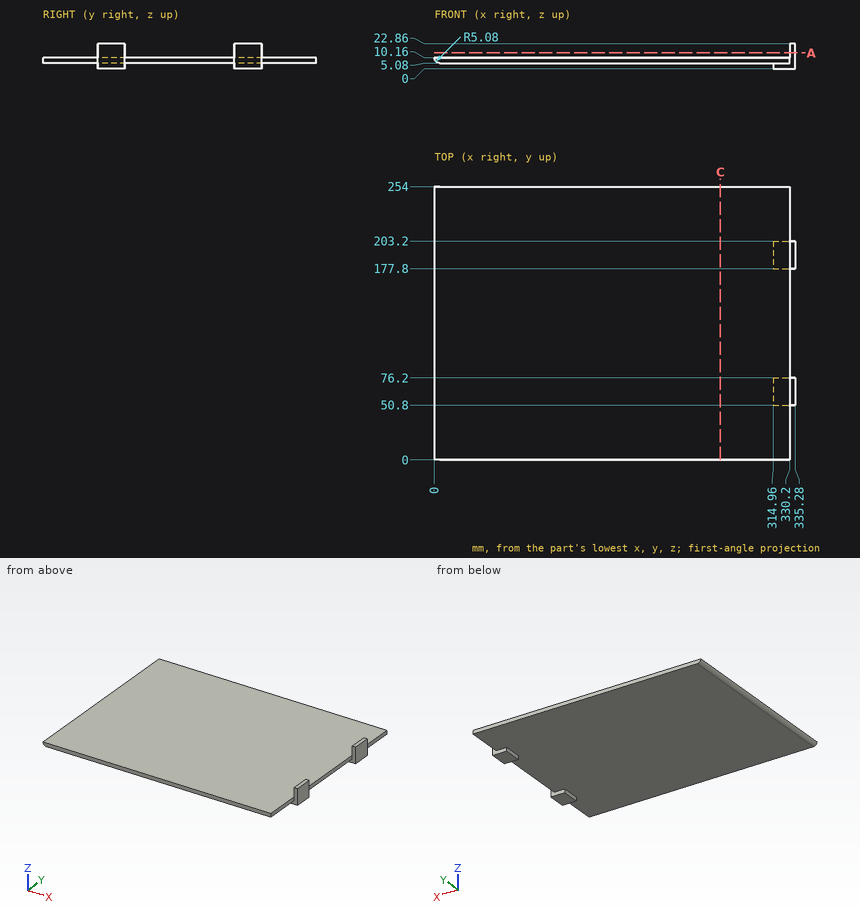
Study the drawing (mm; zero at the part's minimum x, y, z) and answer. Round coordinates to 2 decimals unless told otherwise and drop trailing zeros. Order: outer loops, then holes, each group sorted by start corner. A loop starts at its lowest first (then second) coordinate and runs counter-clockwise, first axis right, second up. Notation, with made-up numbers: (52.5, 57) - (96.5, 57) arc R19 cw to (96.5, 81) - close; hole circle Ø4 at (16, 75.5). An arc over 180 degrees is marked (long way). Use one line per item in the form item = value. Start each with the question number.
(1) Flat-ended cylindrical pins translate along their axes: pin 1 Ø4 at (y, z) = (89.5, 8.5) entering from -X; pin 2 Ø4 at (y, z) = (216.5, 9) entering from +X; pin 3 Ø3 at (x, y) = (40, 136.5) entering from -Z; pin 4 Ø4 at (y, z) = (185, 3) entering from -X. Find the tip coordinate at first contact, or state that the pin passes through.
(2) Find the intervals of material crossed by line 1 along X through (y, z) = (181, 15.5); line 2 along Z through (x, y) = (224, 44); line 3 along X through (y, z) = (75, 4), in increasing order. Write a range as from..to.
(3) The part is cut by section C-C (x = 266). Give the vertices of the cut face in (y, z).
(4) The part is cut by section A-A (z = 14.5). Give the vertices of the cut face in (x, y), then the cut area to 3 significant figures.
Checked values:
q1.pin_1 = 0
q1.pin_2 = 330.2
q1.pin_3 = 5.08
q1.pin_4 = 314.96
q2.line_1 = 330.2..335.28
q2.line_2 = 5.08..10.16
q2.line_3 = 314.96..335.28
q3.outline = (0, 5.08) - (254, 5.08) - (254, 10.16) - (0, 10.16) - close
q4.outline = (330.2, 50.8) - (335.28, 50.8) - (335.28, 76.2) - (330.2, 76.2) - close; (330.2, 177.8) - (335.28, 177.8) - (335.28, 203.2) - (330.2, 203.2) - close
q4.area = 258 mm^2
